Geometry check sheet. Reference: the model listing, model coordinates, mm. Round coordinates to 2 decimals unless told otherwise and drop trailing zeros. Write each loop counter-clockwise with the first axis right and the second up, starting at its lowest first coordinate (ties: lowest second). Pieces come first, ordered by that corner, then holes. Notation, with made-up numbers: (74.5, 36.25) -> (99.5, 36.25) arc R25 cw to (99.5, 66.25) -> close; hole circle Ø9 at (58.25, 87.25). An arc over 180 degrees is marked (long way). Put each result on its own line as item: value. Start each with the question number.
from build123d import *

# Parameters (mm, degrees)
F3_DEPTH = 45.001
F5_DEPTH = 45.001
F6_COUNT = 12
F7_COUNT = 12


with BuildPart() as f1:
    # F0 (on Front) → F1 (revolve)
    with BuildSketch(Plane.XZ):
        Polygon((-3, 0), (0, 0), (0, 45), (-3, 45), (-4, 43.2679491924), (-4, 1.7320508076), align=None)
    revolve(axis=Axis((0, 0, 22.5), (0, 0, -1)))

    # F2 (on face) → F3 (cut, through all)
    with BuildSketch(Plane.XY.offset(45)):
        with BuildLine():
            Line((-3, 0), (-3, 5))
            ThreePointArc((-3, 5), (-5.8309518948, 0), (-3, -5))
            Line((-3, -5), (-3, 0))
        make_face()
        with BuildLine():
            ThreePointArc((5.8309518948, 0), (5.0740937952, 2.8729030888), (3, 5))
            Line((3, 5), (3, 0))
            Line((3, 0), (3, -5))
            ThreePointArc((3, -5), (5.0740937952, -2.8729030888), (5.8309518948, 0))
        make_face()
    extrude(amount=-F3_DEPTH, mode=Mode.SUBTRACT)

    # F4 (on face) → F5 (cut, through all)
    with BuildSketch(Plane.XY.offset(45)):
        Polygon((0.813057266, 4.9082564943), (-0.813057266, 4.9082564943), (0, 3.5), align=None)
        Polygon((0.813057266, -4.9082564943), (0, -3.5), (-0.813057266, -4.9082564943), align=None)
    f5 = extrude(amount=-F5_DEPTH, mode=Mode.SUBTRACT)

    # F6: F5 ×12 about axis
    f6_axis = Axis((0, 0, 45), (0, 0, -1))
    for i in range(1, F6_COUNT):
        add(f5.solids().sort_by_distance((0.406529, 4.204128, 22.4995))[0].rotate(f6_axis, i * 360 / F6_COUNT), mode=Mode.SUBTRACT)

    # F7: F5 ×12 about axis
    f7_axis = Axis((0, 0, 45), (0, 0, 1))
    for i in range(1, F7_COUNT):
        add(f5.solids().sort_by_distance((0.406529, -4.204128, 22.4995))[0].rotate(f7_axis, i * 360 / F7_COUNT), mode=Mode.SUBTRACT)


solid = f1.part
(1) Material ranges on L1, parallel to X at y = -3.25, z = 31; L2, parallel to Y at x = 2.25, z = 6; L3, parallel to X at y = 3, z = 16.5, recorded low to high. Write a range as from..to.
(2) Go/stop test with flat-tipped pins: pin 1 Ø0.5 at (y, z) = (3.5, 29) entering from +X; pin 2 Ø0.6 at (y, z) = (-3, 18.5) entering from -X. Record where each tip stops, or that it passes through.
(3) Sectioned sample at A-A (z = 4.5). Record the cut outline in (x, y).
Found:
1. L1: -2.33..-2.13, -1.75..1.75, 2.13..2.33
1. L2: -3.31..3.31
1. L3: -2.65..2.65
2. pin 1: x = 2.33
2. pin 2: x = -2.95
3. outline: (-3, -2.65) arc R4 ccw to (-2.24, -3.31) -> (-1.75, -3.03) -> (-1.75, -3.6) arc R4 ccw to (-0.28, -3.99) -> (0, -3.5) -> (0.28, -3.99) arc R4 ccw to (1.75, -3.6) -> (1.75, -3.03) -> (2.24, -3.31) arc R4 ccw to (3, -2.65) -> (3, 2.65) arc R4 ccw to (2.24, 3.31) -> (1.75, 3.03) -> (1.75, 3.6) arc R4 ccw to (0.28, 3.99) -> (0, 3.5) -> (-0.28, 3.99) arc R4 ccw to (-1.75, 3.6) -> (-1.75, 3.03) -> (-2.24, 3.31) arc R4 ccw to (-3, 2.65) -> close
